Part model, mm, in its own coordinate system. A direction names the side the tool comes from. Coordinates: 2 decimals unless noted, no trailing zeros. Loops run counter-clockwise (first coordinate to the right, second up) from the corner with the lowest first, then second, coordinate; pieces in that order, holes last. Notation, with made-up numbers: (43.5, 1.5) -> (63.5, 1.5) arc R21 ccw to (63.5, 25.5) -> close; hole circle Ø8 at (21, -23.75). An arc over 180 degrees is marked (long way). One line per question, with ' | ' between items. Start each with the question number.
1) Cut at B-B (x = 1.6). Count the separate pieces of the cut face and the enclosed holes in it, plus the area to 3 significant figures.
2) Drop flat-ended pins along their axis: pin 1 (1.5 mm diameter, centred on x = 1, y = 8.5, fed in from +Z); pin 2 (1.5 mm diameter, centred on x = 1, y = 20, fed in from +Z). Give the stop position or say it passes through.
3) Probe L1, parallel to Y at x = 0.8, z = 0; L2, parallel to Y at x = 1.8, z = -16.5; L3, parallel to Y at x = 0.25, z = 10. List the from-to ranges inside material, lowest first. Write a range as from..to.
4) 3-axis set-ups, long thin cutter, end or side, ignore diameter. For faces 1 (the face through (2.54, -5, -10)), 2 (the face through (1.25, 13.7, 5.15)): which of +Z, -Z, +X, -X, +Y, -Y reach the whole face in a straight line?
5) Two-plate mould, pull along Z, no slides. Class faces 3 (the face through (0, -5, -10)), 4 (the face through (1.252, 19.817, -8.033)): released by +Z, released by -Z, zero draft, split by the parting line, or undercut.
6) Cut at D-D (z = -13.5). List the corners of the cut face in (x, y).
7) Cut at A-A (z = 0). List the corners of the cut face in (x, y).
from build123d import *

# Parameters (mm, degrees)
SKETCH1_R           = 25.4
SKETCH1_R_2         = 2.126996
SKETCH1_R_3         = 10.925995089
BOSS_EXTRUDE1_DEPTH = 2.54
FILLET1_R           = 5.08


with BuildPart() as part:
    # Sketch1 → Boss-Extrude1 (new body)
    with BuildSketch(Plane(origin=(0, 0, 0), x_dir=(0, 0, -1), z_dir=(1, 0, 0))):
        Circle(SKETCH1_R)
        with Locations((0, 21.9999941)):
            Circle(SKETCH1_R_2, mode=Mode.SUBTRACT)
        with Locations((14.999999972, 0)):
            Circle(SKETCH1_R_2, mode=Mode.SUBTRACT)
        with Locations((21.9999941, 0)):
            Circle(SKETCH1_R_2, mode=Mode.SUBTRACT)
        with Locations((0, -21.9999941)):
            Circle(SKETCH1_R_2, mode=Mode.SUBTRACT)
        with Locations((-21.9999941, 0)):
            Circle(SKETCH1_R_2, mode=Mode.SUBTRACT)
        with Locations((0, -14.999999972)):
            Circle(SKETCH1_R_2, mode=Mode.SUBTRACT)
        with Locations((-14.999999972, 0)):
            Circle(SKETCH1_R_2, mode=Mode.SUBTRACT)
        with Locations((0, 14.999999972)):
            Circle(SKETCH1_R_2, mode=Mode.SUBTRACT)
        Circle(SKETCH1_R_3, mode=Mode.SUBTRACT)
        with BuildLine():
            Line((12.944345277, 3.71173128), (21.974442369, 6.301069954))
            ThreePointArc((21.974442369, 6.301069954), (16.164461018, 16.164461018), (6.301069954, 21.974442369))
            Line((6.301069954, 21.974442369), (3.71173128, 12.944345277))
            ThreePointArc((3.71173128, 12.944345277), (9.521896443, 9.521896443), (12.944345277, 3.71173128))
        make_face(mode=Mode.SUBTRACT)
        with BuildLine():
            Line((-12.944345277, 3.71173128), (-21.974442369, 6.301069954))
            ThreePointArc((-21.974442369, 6.301069954), (-16.164461018, 16.164461018), (-6.301069954, 21.974442369))
            Line((-6.301069954, 21.974442369), (-3.71173128, 12.944345277))
            ThreePointArc((-3.71173128, 12.944345277), (-9.521896443, 9.521896443), (-12.944345277, 3.71173128))
        make_face(mode=Mode.SUBTRACT)
        with BuildLine():
            Line((3.71173128, -12.944345277), (6.301069954, -21.974442369))
            ThreePointArc((6.301069954, -21.974442369), (16.164461018, -16.164461018), (21.974442369, -6.301069954))
            Line((21.974442369, -6.301069954), (12.944345277, -3.71173128))
            ThreePointArc((12.944345277, -3.71173128), (9.521896443, -9.521896443), (3.71173128, -12.944345277))
        make_face(mode=Mode.SUBTRACT)
        with BuildLine():
            Line((-12.944345277, -3.71173128), (-21.974442369, -6.301069954))
            ThreePointArc((-21.974442369, -6.301069954), (-16.164461018, -16.164461018), (-6.301069954, -21.974442369))
            Line((-6.301069954, -21.974442369), (-3.71173128, -12.944345277))
            ThreePointArc((-3.71173128, -12.944345277), (-9.521896443, -9.521896443), (-12.944345277, -3.71173128))
        make_face(mode=Mode.SUBTRACT)
    extrude(amount=BOSS_EXTRUDE1_DEPTH)

    # Fillet1
    # the kernel refuses this fillet: 5.08 mm, written as the material it adds along each edge
    with BuildSketch(Plane(origin=(0, 6.301069954, -21.974442369), x_dir=(0, 0.911397711724722, 0.41152668329397635), z_dir=(1, 0, 0)), Plane(origin=(0, -21.974442369, -6.301069954), x_dir=(0, 0.4115266832939732, -0.9113977117247234), z_dir=(1, 0, 0)), Plane(origin=(0, -6.301069954, 21.974442369), x_dir=(0, -0.9113977117247248, -0.4115266832939699), z_dir=(1, 0, 0))) as fillet1_piece_1:
        with BuildLine():
            CenterArc((5.867179819, 5.026781091), FILLET1_R, 171.6992252, 106.601549599)
            Line((0.840398727, 5.760178569), (0, 0))
            ThreePointArc((0, 0), (3.300288648, -0.239485089), (6.600577296, 0))
        make_face()
    extrude(amount=2.54)
    with BuildSketch(Plane(origin=(0, 3.71173128, -12.944345277), x_dir=(0, 0.9139096848416328, 0.4059175876365389), z_dir=(1, 0, 0))) as fillet1_piece_2:
        with BuildLine():
            CenterArc((4.426790217, -5.031193515), FILLET1_R, 97.948640691, 74.102718618)
            Line((-0.604403297, -4.328703786), (0, 0))
            ThreePointArc((0, 0), (1.862150244, -0.12937557), (3.724300488, 0))
        make_face()
    extrude(amount=2.54)
    with BuildSketch(Plane(origin=(0, 12.944345277, -3.71173128), x_dir=(0, -0.40591758763655106, -0.9139096848416274), z_dir=(1, 0, 0)), Plane(origin=(0, -12.944345277, 3.71173128), x_dir=(0, 0.4059175876365596, 0.9139096848416237), z_dir=(1, 0, 0)), Plane(origin=(0, 3.71173128, 12.944345277), x_dir=(0, 0.9139096848416286, -0.4059175876365486), z_dir=(1, 0, 0))) as fillet1_piece_3:
        with BuildLine():
            CenterArc((4.426790217, 5.031193515), FILLET1_R, 187.948640691, 74.102718618)
            Line((-0.604403297, 4.328703786), (0, 0))
            ThreePointArc((0, 0), (1.862150244, 0.12937557), (3.724300488, 0))
        make_face()
    extrude(amount=2.54)
    with BuildSketch(Plane(origin=(0, 21.974442369, -6.301069954), x_dir=(0, -0.9612616959383177, 0.275637355817003), z_dir=(1, 0, 0)), Plane(origin=(0, -6.301069954, -21.974442369), x_dir=(0, 0.2756373558170063, 0.9612616959383169), z_dir=(1, 0, 0)), Plane(origin=(0, 6.301069954, 21.974442369), x_dir=(0, -0.27563735581699955, -0.9612616959383188), z_dir=(1, 0, 0))) as fillet1_piece_4:
        with BuildLine():
            CenterArc((5.821162011, 5.08), FILLET1_R, 163.398450401, 106.601549599)
            ThreePointArc((0.952922586, 6.531428571), (0.239485089, 3.300288648), (0, 0))
            Line((0, 0), (5.821162011, 0))
        make_face()
    extrude(amount=2.54)
    with BuildSketch(Plane(origin=(0, -3.71173128, -12.944345277), x_dir=(0, -0.2756373558170063, -0.9612616959383169), z_dir=(1, 0, 0))) as fillet1_piece_5:
        with BuildLine():
            CenterArc((4.370695575, -5.08), FILLET1_R, 90, 74.102718618)
            ThreePointArc((-0.515016307, -3.688518989), (-0.12937557, -1.862150244), (0, 0))
            Line((0, 0), (4.370695575, 0))
        make_face()
    extrude(amount=2.54)
    with BuildSketch(Plane(origin=(0, -12.944345277, -3.71173128), x_dir=(0, -0.9612616959383224, -0.2756373558169866), z_dir=(1, 0, 0)), Plane(origin=(0, -3.71173128, 12.944345277), x_dir=(0, -0.27563735581698295, 0.9612616959383236), z_dir=(1, 0, 0)), Plane(origin=(0, 12.944345277, 3.71173128), x_dir=(0, 0.9612616959383206, 0.2756373558169933), z_dir=(1, 0, 0))) as fillet1_piece_6:
        with BuildLine():
            CenterArc((4.370695575, 5.08), FILLET1_R, 195.897281382, 74.102718618)
            ThreePointArc((-0.515016307, 3.688518989), (-0.12937557, 1.862150244), (0, 0))
            Line((0, 0), (4.370695575, 0))
        make_face()
    extrude(amount=2.54)
    with BuildSketch(Plane(origin=(0, -21.974442369, 6.301069954), x_dir=(0, 0.41152668329399555, 0.9113977117247133), z_dir=(1, 0, 0))) as fillet1_piece_7:
        with BuildLine():
            CenterArc((5.867179819, -5.026781091), FILLET1_R, 81.6992252, 106.601549599)
            Line((0.840398727, -5.760178569), (0, 0))
            ThreePointArc((0, 0), (3.300288648, 0.239485089), (6.600577296, 0))
        make_face()
    extrude(amount=2.54)
    with BuildSketch(Plane(origin=(0, 21.974442369, 6.301069954), x_dir=(0, -0.9612616959383207, -0.27563735581699317), z_dir=(1, 0, 0))) as fillet1_piece_8:
        with BuildLine():
            CenterArc((5.821162011, -5.08), FILLET1_R, 90, 106.601549599)
            ThreePointArc((0.952922586, -6.531428571), (0.239485089, -3.300288648), (0, 0))
            Line((0, 0), (5.821162011, 0))
        make_face()
    extrude(amount=2.54)


solid = part.part
Reported:
1) separate pieces: 1 | enclosed holes: 13 | area: 942 mm²
2) pin 1: stops at z = 24.19 | pin 2: stops at z = 16.57
3) L1: y = -25.4..-24.13, -19.87..-17.13, -12.87..-10.93, 10.93..12.87, 17.13..19.87, 24.13..25.4 | L2: y = -19.31..-15.82, -4.78..-1.51, 1.51..4.78, 15.82..19.31 | L3: y = -23.35..-20.04, -9.02..-4.4, 4.4..9.02, 20.04..23.35
4) face 1: +Z, -Z, +X, +Y, -Y | face 2: +X, -X
5) face 3: zero draft | face 4: undercut
6) outline: (0, -21.52) -> (2.54, -21.52) -> (2.54, -18.45) -> (0, -18.45) -> close; (0, -5.24) -> (2.54, -5.24) -> (2.54, -1.51) -> (0, -1.51) -> close; (0, 1.51) -> (2.54, 1.51) -> (2.54, 5.24) -> (0, 5.24) -> close; (0, 18.45) -> (2.54, 18.45) -> (2.54, 21.52) -> (0, 21.52) -> close
7) outline: (0, -25.4) -> (2.54, -25.4) -> (2.54, -24.13) -> (0, -24.13) -> close; (0, -19.87) -> (2.54, -19.87) -> (2.54, -17.13) -> (0, -17.13) -> close; (0, -12.87) -> (2.54, -12.87) -> (2.54, -10.93) -> (0, -10.93) -> close; (0, 10.93) -> (2.54, 10.93) -> (2.54, 12.87) -> (0, 12.87) -> close; (0, 17.13) -> (2.54, 17.13) -> (2.54, 19.87) -> (0, 19.87) -> close; (0, 24.13) -> (2.54, 24.13) -> (2.54, 25.4) -> (0, 25.4) -> close
